Autodesk Inventor part; units mm, degrees
ref_plane "YZ Plane" through (0, 0, 0) normal (1, 0, 0) x (0, 1, 0)
ref_plane "XZ Plane" through (0, 0, 0) normal (0, 1, 0) x (-1, 0, 0)
ref_plane "XY Plane" through (0, 0, 0) normal (0, 0, 1) x (1, 0, 0)
sketch "Sketch1" plane through (0, 0, 0) normal (0, 0, 1) x (1, 0, 0)
  line L0 (0, 0) -> (68, 0)
  line L1 (68, 0) -> (68, 68)
  line L2 (68, 68) -> (0, 68)
  line L3 (0, 68) -> (0, 0)
  dimension "d1" = 68
  dimension "d2" = 68
extrude "Extrusion1" add sketch "Sketch1" along normal blind 480
sketch "Sketch2" plane through (0, 0, 480) normal (0, 0, 1) x (1, 0, 0)
  line L0 (10, 58) -> (58, 58)
  line L1 (58, 58) -> (58, 10)
  line L2 (58, 10) -> (10, 10)
  line L3 (10, 10) -> (10, 58)
  line L4 (68, 68) -> (0, 68)
  line L5 (0, 68) -> (0, 0)
  line L6 (0, 0) -> (68, 0)
  line L7 (68, 0) -> (68, 68)
  dimension "d5" = 10
  dimension "d6" = 10
  dimension "d7" = 10
  dimension "d8" = 10
extrude "Extrusion2" cut sketch "Sketch2" against normal blind 900 contours L0 L1 L2 L3
sketch "Sketch3" plane through (68, 0, 0) normal (1, 0, 0) x (0, 0, -1)
  line L0 (-470, 58) -> (-10, 58)
  line L1 (-10, 58) -> (-10, 10)
  line L2 (-10, 10) -> (-470, 10)
  line L3 (-470, 10) -> (-470, 58)
  line L4 (0, 68) -> (-480, 68)
  line L5 (-480, 0) -> (-480, 68)
  line L6 (0, 0) -> (-480, 0)
  line L7 (0, 0) -> (0, 68)
  dimension "d11" = 10
  dimension "d12" = 10
  dimension "d13" = 10
  dimension "d14" = 10
extrude "Extrusion3" cut sketch "Sketch3" against normal blind 900 contours L0 L1 L2 L3
sketch "Sketch4" plane through (0, 68, 0) normal (0, 1, 0) x (1, 0, 0)
  line L0 (68, -10) -> (58, -10)
  line L1 (10, -480) -> (10, -470)
  line L2 (58, -10) -> (10, -10)
  line L3 (10, -10) -> (10, -470)
  line L4 (10, -470) -> (58, -470)
  line L5 (58, -470) -> (58, -10)
  point P0 (0, 0)
extrude "Extrusion4" cut sketch "Sketch4" against normal blind 900
sketch "Sketch5" plane through (0, 0, 480) normal (0, 0, 1) x (1, 0, 0)
  line L0 (68, 68) -> (0, 68)
  line L1 (0, 0) -> (68, 0)
  line L2 (0, 68) -> (68, 68)
  line L3 (68, 68) -> (68, 0)
  line L4 (68, 0) -> (0, 0)
  line L5 (0, 0) -> (0, 68)
  line L6 (10, 58) -> (0, 58)
  line L7 (58, 58) -> (58, 10)
  line L8 (10, 58) -> (58, 58)
  line L9 (58, 58) -> (58, 10)
  line L10 (58, 10) -> (10, 10)
  line L11 (10, 10) -> (10, 58)
extrude "Extrusion5" add sketch "Sketch5" along normal blind 10
sketch "Sketch6" plane through (0, 68, 0) normal (0, 1, 0) x (1, 0, 0)
  line L0 (58, -490) -> (58, -470)
  line L1 (10, -490) -> (10, -470)
  line L2 (58, -470) -> (10, -470)
  line L3 (10, -470) -> (10, -480)
  line L4 (10, -480) -> (58, -480)
  line L5 (58, -480) -> (58, -470)
  point P0 (0, 0)
extrude "Extrusion6" cut sketch "Sketch6" against normal blind 900
sketch "Sketch7" plane through (68, 0, 0) normal (1, 0, 0) x (0, 0, -1)
  line L0 (-470, 10) -> (-470, 58)
  line L1 (-480, 10) -> (-480, 0)
  line L2 (-470, 58) -> (-480, 58)
  line L3 (-480, 58) -> (-480, 10)
  line L4 (-480, 10) -> (-470, 10)
  line L5 (-470, 10) -> (-470, 58)
  point P0 (0, 0)
extrude "Extrusion7" cut sketch "Sketch7" against normal blind 900
sketch "Sketch8" plane through (0, 0, 0) normal (0, 0, -1) x (-1, 0, 0)
  line L0 (-68, 0) -> (-68, 68)
  line L1 (-68, 68) -> (0, 68)
  line L2 (0, 68) -> (0, 0)
  line L3 (0, 0) -> (-68, 0)
  line L4 (-68, 0) -> (-68, 68)
  line L5 (-58, 58) -> (-10, 58)
  line L6 (-10, 58) -> (-10, 10)
  line L7 (-10, 10) -> (-58, 10)
  line L8 (-58, 10) -> (-58, 58)
extrude "Extrusion8" add sketch "Sketch8" along normal blind 10
sketch "Sketch9" plane through (0, 68, 490) normal (0, 1, 0) x (1, 0, 0)
  line L0 (10, 480) -> (10, 500)
  line L1 (58, 480) -> (58, 500)
  line L2 (10, 480) -> (58, 480)
  line L3 (58, 480) -> (58, 490)
  line L4 (58, 490) -> (10, 490)
  line L5 (10, 490) -> (10, 480)
  point P0 (0, 490)
extrude "Extrusion9" cut sketch "Sketch9" against normal blind 900
sketch "Sketch10" plane through (68, 0, 490) normal (1, 0, 0) x (0, 0, -1)
  line L0 (10, 58) -> (480, 58)
  line L1 (490, 10) -> (500, 10)
  line L2 (480, 58) -> (490, 58)
  line L3 (490, 58) -> (490, 10)
  line L4 (490, 10) -> (480, 10)
  line L5 (480, 10) -> (480, 58)
  point P0 (490, 0)
extrude "Extrusion10" cut sketch "Sketch10" against normal blind 900
sketch "Sketch11" plane through (68, 0, 490) normal (1, 0, 0) x (0, 0, -1)
  line L0 (0, 68) -> (0, 0)
  line L1 (500, 0) -> (500, 68)
  line L2 (0, 68) -> (500, 68)
  line L3 (500, 68) -> (500, 0)
  line L4 (500, 0) -> (0, 0)
  line L5 (0, 0) -> (0, 68)
  line L6 (490, 58) -> (490, 10)
  line L7 (10, 58) -> (490, 58)
  line L8 (490, 58) -> (490, 10)
  line L9 (490, 10) -> (10, 10)
  line L10 (10, 10) -> (10, 58)
  point P0 (490, 0)
extrude "Extrusion11" add sketch "Sketch11" along normal blind 20
sketch "Sketch12" plane through (0, 68, 490) normal (0, 1, 0) x (1, 0, 0)
  line L0 (58, 10) -> (58, 490)
  line L1 (88, 490) -> (58, 490)
  line L2 (58, 10) -> (78, 10)
  line L3 (78, 10) -> (78, 490)
  line L4 (78, 490) -> (58, 490)
  line L5 (58, 490) -> (58, 10)
  point P0 (0, 490)
  dimension "d33" = 20
extrude "Extrusion12" cut sketch "Sketch12" against normal blind 900
sketch "Sketch13" plane through (0, 0, -10) normal (0, 0, -1) x (-1, 0, 0)
  line L0 (-58, 58) -> (-10, 58)
  line L1 (-58, 58) -> (-78, 58)
  line L2 (-78, 58) -> (-78, 10)
  line L3 (-78, 10) -> (-58, 10)
  line L4 (-58, 10) -> (-58, 58)
  point P0 (0, 0)
  dimension "d36" = 20
extrude "Extrusion13" cut sketch "Sketch13" against normal blind 900
sketch "Sketch14" plane through (0, 68, 490) normal (0, 1, 0) x (1, 0, 0)
  line L0 (0, 0) -> (88, 0)
  line L1 (0, 500) -> (88, 500)
  line L2 (0, 0) -> (88, 0)
  line L3 (88, 0) -> (88, 500)
  line L4 (88, 500) -> (0, 500)
  line L5 (0, 500) -> (0, 0)
  line L6 (10, 10) -> (10, 490)
  line L7 (78, 10) -> (78, 490)
  line L8 (10, 10) -> (78, 10)
  line L9 (78, 10) -> (78, 490)
  line L10 (78, 490) -> (10, 490)
  line L11 (10, 490) -> (10, 10)
  point P0 (0, 490)
extrude "Extrusion14" add sketch "Sketch14" along normal blind 10
sketch "Sketch15" plane through (88, 0, 490) normal (1, 0, 0) x (0, 0, -1)
  line L0 (10, 58) -> (490, 58)
  line L1 (490, 78) -> (490, 58)
  line L2 (10, 58) -> (490, 58)
  line L3 (490, 58) -> (490, 68)
  line L4 (490, 68) -> (10, 68)
  line L5 (10, 68) -> (10, 58)
  point P0 (490, 0)
extrude "Extrusion15" cut sketch "Sketch15" against normal blind 900
sketch "Sketch16" plane through (0, 0, -10) normal (0, 0, -1) x (-1, 0, 0)
  line L0 (-78, 10) -> (-78, 58)
  line L1 (-10, 68) -> (0, 68)
  line L2 (-78, 58) -> (-10, 58)
  line L3 (-10, 58) -> (-10, 68)
  line L4 (-10, 68) -> (-78, 68)
  line L5 (-78, 68) -> (-78, 58)
  point P0 (0, 0)
extrude "Extrusion16" cut sketch "Sketch16" against normal blind 900
sketch "Sketch17" plane through (0, 78, 490) normal (0, 1, 0) x (1, 0, 0)
  line L0 (88, 0) -> (88, 500)
  line L1 (0, 0) -> (88, 0)
  line L2 (88, 500) -> (0, 500)
  line L3 (0, 500) -> (0, 0)
  line L4 (0, 0) -> (88, 0)
  line L5 (88, 0) -> (88, 500)
  line L6 (78, 490) -> (78, 10)
  line L7 (10, 10) -> (10, 490)
  line L8 (78, 490) -> (10, 490)
  line L9 (10, 490) -> (10, 10)
  line L10 (10, 10) -> (78, 10)
  line L11 (78, 10) -> (78, 490)
  point P0 (0, 490)
extrude "Extrusion17" add sketch "Sketch17" along normal blind 20
sketch "Sketch18" plane through (88, 0, 490) normal (1, 0, 0) x (0, 0, -1)
  line L0 (490, 68) -> (10, 68)
  line L1 (10, 68) -> (490, 68)
  line L2 (490, 68) -> (490, 88)
  line L3 (490, 88) -> (10, 88)
  line L4 (10, 88) -> (10, 68)
  point P0 (490, 0)
  dimension "d47" = 20
extrude "Extrusion18" cut sketch "Sketch18" against normal blind 900
sketch "Sketch19" plane through (0, 0, 490) normal (0, 0, 1) x (1, 0, 0)
  line L0 (10, 68) -> (10, 10)
  line L1 (78, 88) -> (78, 98)
  line L2 (10, 68) -> (78, 68)
  line L3 (78, 68) -> (78, 88)
  line L4 (78, 88) -> (10, 88)
  line L5 (10, 88) -> (10, 68)
  point P0 (0, 0)
extrude "Extrusion19" cut sketch "Sketch19" against normal blind 900
sketch "Sketch20" plane through (0, 0, -10) normal (-1, 0, 0) x (0, 0, 1)
  line L0 (0, 98) -> (500, 98)
  line L1 (0, 98) -> (500, 98)
  line L2 (500, 98) -> (500, 0)
  line L3 (500, 0) -> (0, 0)
  line L4 (0, 0) -> (0, 98)
  line L5 (10, 88) -> (490, 88)
  line L6 (490, 10) -> (10, 10)
  line L7 (10, 88) -> (490, 88)
  line L8 (490, 88) -> (490, 10)
  line L9 (490, 10) -> (10, 10)
  line L10 (10, 10) -> (10, 88)
  point P0 (10, 0)
extrude "Extrusion20" add sketch "Sketch20" along normal blind 10
sketch "Sketch21" plane through (0, 0, 490) normal (0, 0, 1) x (1, 0, 0)
  line L0 (78, 88) -> (10, 88)
  line L1 (10, 10) -> (-10, 10)
  line L2 (10, 88) -> (0, 88)
  line L3 (0, 88) -> (0, 10)
  line L4 (0, 10) -> (10, 10)
  line L5 (10, 10) -> (10, 88)
  point P0 (0, 0)
extrude "Extrusion21" cut sketch "Sketch21" against normal blind 900
sketch "Sketch22" plane through (0, 98, 490) normal (0, 1, 0) x (1, 0, 0)
  line L0 (10, 490) -> (78, 490)
  line L1 (0, 10) -> (-10, 10)
  line L2 (10, 490) -> (0, 490)
  line L3 (0, 490) -> (0, 10)
  line L4 (0, 10) -> (10, 10)
  line L5 (10, 10) -> (10, 490)
  point P0 (0, 490)
extrude "Extrusion22" cut sketch "Sketch22" against normal blind 900
sketch "Sketch24" plane through (-10, 0, -10) normal (-1, 0, 0) x (0, 0, 1)
  line L0 (500, 0) -> (0, 0)
  line L1 (10, 88) -> (10, 10)
  line L2 (0, 0) -> (10, 0)
  line L3 (10, 0) -> (10, 10)
  line L4 (10, 10) -> (0, 10)
  line L5 (0, 10) -> (0, 0)
  point P0 (10, 0)
extrude "Extrusion24" add sketch "Sketch24" along normal blind 64.455
properties part number "Accumalator Housing"
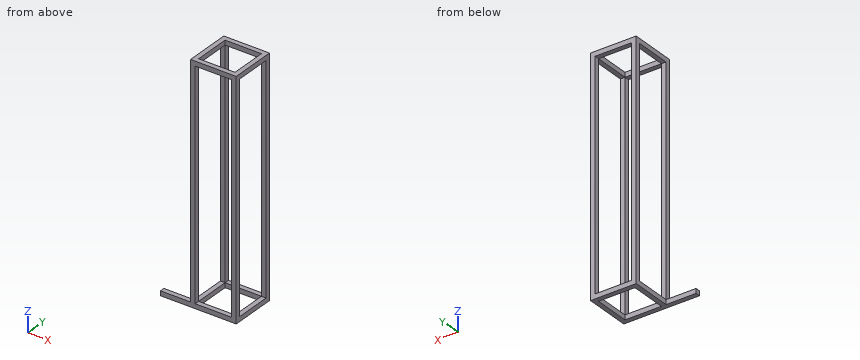
Can you work these out from the model? Positions are in its coordinate system, mm. Round coordinates to 2 decimals unless told otherwise and drop trailing zeros. Loops run counter-clockwise (first coordinate to the right, second up) from the corner with the lowest first, then second, coordinate; pieces in that order, holes last. Notation, with made-up numbers: M 24,56 L 69,56 A34 ccw 69,90 Z; hole C -1.75,86 d1. An arc over 180 degrees is marked long. Write item = value, one per line. Start each with the question number.
(1) Suppose I cut it at C-C on x = -60. Write out the boundary of the cut face in (y, z), plus the area to 3 significant figures.
(2) Suppose I cut it at A-A on y = 44. Write out the boundary of the cut face in (x, z), plus the area to 3 significant figures.
(3) I'm going to push flat-ended pins straight in: P1, Ø3, axis at x = -39, z = -4, coming from the +Y side; P2, Ø3, axis at x = 25.5, y = 87.5, coming from the +Z side; P3, Ø8, axis at y = 93.5, z = 306.5, coming from the -X side; P4, Ø5, axis at x = -49, y = 4.5, coming from the +Z side. Where does each tip first touch, or does it pass through?
(4) I need wall thicknesses on line 1 along X through (y, z) = (8.5, 166); line 2 along Z through (x, y) = (28.5, 9); line 3 along Z through (x, y) = (-52, 7). Which ranges of each line are inside material? Lowest first, please.
(5) Suppose I cut it at B-B on x = 27. Write out the boundary of the cut face in (y, z).
Answer block:
q1.outline = M 0,-10 L 10,-10 L 10,0 L 0,0 Z
q1.area = 100 mm²
q2.outline = M -10,-10 L 0,-10 L 0,0 L -10,0 Z; M -10,480 L 0,480 L 0,490 L -10,490 Z; M 78,-10 L 88,-10 L 88,0 L 78,0 Z; M 78,480 L 88,480 L 88,490 L 78,490 Z
q2.area = 400 mm²
q3.P1 = 10
q3.P2 = 490
q3.P3 = -10
q3.P4 = 0
q4.line_1 = -10 to 0, 78 to 88
q4.line_2 = -10 to 0, 480 to 490
q4.line_3 = -10 to 0
q5.outline = M 0,-10 L 10,-10 L 10,0 L 0,0 Z; M 0,480 L 10,480 L 10,490 L 0,490 Z; M 88,-10 L 98,-10 L 98,0 L 88,0 Z; M 88,480 L 98,480 L 98,490 L 88,490 Z
